Autodesk Inventor part; units mm, degrees
ref_plane "Work Plane2" through (-55.063, 1219.2, 61.6037) normal (-0.9994, -0.0355, 0) x (0, 0, -1)
ref_plane "Work Plane3" through (-184.9668, 1219.2, -13.3963) normal (0.4997, -0.0355, -0.8655) x (0.866, 0, 0.5)
ref_plane "Work Plane4" through (-55.063, 1219.2, -88.3963) normal (0.4997, -0.0355, 0.8655) x (-0.866, 0, 0.5)
sketch "Sketch1" plane through (0, 0, 0) normal (0, 1, 0) x (-1, 0, 0)
  line L0 (11.7617, 136.6037) -> (11.7617, -163.3963)
  line L1 (11.7617, -163.3963) -> (271.5693, -13.3963)
  line L2 (271.5693, -13.3963) -> (11.7617, 136.6037)
  circle A0 centre (98.3643, -13.3963) radius 86.6025
  line L3 (55.063, 61.6037) -> (55.063, -88.3963)
  line L4 (55.063, 61.6037) -> (184.9668, -13.3963)
  line L5 (55.063, 61.6037) -> (205.063, 61.6037) construction
  line L6 (184.9668, -13.3963) -> (55.063, -88.3963)
  circle A1 centre (98.3643, -13.3963) radius 43.3013
  point P0 (85.0813, -150)
  point P1 (141.6655, 61.6037)
  point P2 (141.6655, -88.3963)
  point P3 (11.7617, -13.3963)
  point P4 (203.5969, -52.6402)
  dimension "d10" = 300
  dimension "d11" = 300
  dimension "d12" = 60
  dimension "d13" = 150
  dimension "d14" = 150
  dimension "d15" = 30
ref_plane "Work Plane1" through (-52.1275, 0, 74.1452) normal (0, -1, 0) x (0, 0, -1)
extrude "Extrusion2" add sketch "Sketch1" along normal blind 1219.2
sketch "Sketch2" plane through (0, 1219.2, 0) normal (0, 1, 0) x (1, 0, 0)
  line L0 (-271.5693, 13.3963) -> (-11.7617, -136.6037)
  line L1 (-11.7617, -136.6037) -> (-11.7617, 163.3963)
  line L2 (-11.7617, 163.3963) -> (-271.5693, 13.3963)
  circle A0 centre (-98.3643, 13.3963) radius 86.6025
  line L3 (-55.063, -61.6037) -> (-55.063, 88.3963)
  line L4 (-55.063, 88.3963) -> (-184.9668, 13.3963)
  line L5 (-184.9668, 13.3963) -> (-55.063, -61.6037)
  circle A1 centre (-98.3643, 13.3963) radius 43.3013
  point P0 (0, 0)
  point P1 (-141.6655, -61.6037)
  point P2 (-11.7617, 13.3963)
  point P3 (-141.6655, 88.3963)
  dimension "d18" = 150
  dimension "d19" = 150
ref_plane "Work Plane2" through (-55.063, 1219.2, 61.6037) normal (-0.9994, -0.0355, 0) x (0, 0, -1)
split "Split1" plane through (-55.063, 1219.2, 61.6037) removes the side toward (0.9994, 0.0355, 0)
ref_plane "Work Plane3" through (-184.9668, 1219.2, -13.3963) normal (0.4997, -0.0355, -0.8655) x (0.866, 0, 0.5)
split "Split2" plane through (-184.9668, 1219.2, -13.3963) removes the side toward (-0.4997, 0.0355, 0.8655)
ref_plane "Work Plane4" through (-55.063, 1219.2, -88.3963) normal (0.4997, -0.0355, 0.8655) x (-0.866, 0, 0.5)
split "Split3" plane through (-55.063, 1219.2, -88.3963) removes the side toward (-0.4997, 0.0355, -0.8655)
extrude "Extrusion3" add sketch "Sketch2" along normal blind 762 contours L4 A1 L5 | L5 A1 L3 | L3 A1 L4 | A1
properties part number "pillar"
Geometry: final body of the model. Coordinates: model frame, mm. A direction names the side the tool comes from. Round coordinates to 2 decimals unless told otherwise and drop trailing zeros. Write each loop counter-clockwise with the first axis right and the second up, starting at its lowest first coordinate (ties: lowest second). Pieces come first, ordered by that corner, then holes.
Item 1: Section query C-C (y = 1030). Return loops of the section in (x, z).
Item 2: Set-up query: faces 1 (the face through (-120.92, 1594.87, 23.58)), 2 (the face through (-119.11, 1594.87, -51.42)), 3 (the face through (-111, 0, -11)), 4 (the face through (-106, 1981.2, -14)), 5 (the face through (-55.063, 1595, -12)). Return all of +Z, -Z, +X, -X, +Y, -Y with unobstructed straight access to the full face (end or side cutting, diameter ignored); none if empty.
Item 3: Pin query (flat end, axial travel): P1, Ø1, axis at y = 983, z = 42.5, coming from the -X side; P2, Ø1, axis at x = -57, y = 363, coming from the +Z side; P3, Ø12, axis at y = 580, z = 88.5, coming from the +X side. Return the tip coordinate at first contact, or that it passes through.
Item 4: Material intervals for L1, parallel to X at y = 799, z = 69; L2, parallel to X at y = 1474, z = -36.5; L3, parallel to Z at x = -86.5, y = 1318.5, sorted ascending.
Item 5: Section query D-D (x = -33). Return loops of the section in (y, z), plus the area to 3 significant figures.
Completed:
1. outline: (-198.41, -13.4) - (-48.34, -100.04) - (-48.34, 73.24) - close
2. face 1: +Z, -X, +Y
2. face 2: -Z, -X, +Y
2. face 3: +Z, -Z, +X, -X, -Y
2. face 4: +Z, -Z, +X, -X, +Y
2. face 5: +Z, -Z, +X, +Y
3. P1: stops at x = -105.8
3. P2: stops at z = 95.89
3. P3: stops at x = -32.14
4. L1: x = -72.11 to -40.14
4. L2: x = -144.95 to -55.06
4. L3: z = -70.25 to 43.45
5. outline: (0, -151.13) - (0.19, -151.13) - (598.08, -126.61) - (598.08, 99.82) - (0.2, 124.34) - (0, 124.34) - close
5. area: 150,000 mm2
